```python
from build123d import *

# Parameters (mm, degrees)
SKETCH1_R                = 6.5
BOSS_EXTRUDE1_DEPTH      = 20
SKETCH2_R                = 6.45
BOSS_EXTRUDE2_DEPTH      = 9
SKETCH3_R                = 4
BOSS_EXTRUDE3_DEPTH      = 3
SKETCH4_RX               = 10
SKETCH4_RY               = 8
BOSS_EXTRUDE4_DEPTH      = 4
BOSS_EXTRUDE4_DEPTH_BACK = 4
FILLET2_R                = 1
SKETCH5_R                = 2
BOSS_EXTRUDE5_DEPTH      = 11.5
SKETCH8_R                = 2.5
CUT_EXTRUDE1_DEPTH       = 11.5
SKETCH9_R                = 6.45
BOSS_EXTRUDE6_DEPTH      = 60
SKETCH10_R               = 2
CUT_EXTRUDE2_DEPTH       = 10
SKETCH11_R               = 3.674860137
SKETCH11_R_2             = 2
BOSS_EXTRUDE7_DEPTH      = 1


with BuildPart() as part:
    # Sketch1 → Boss-Extrude1 (new body)
    with BuildSketch(Plane(origin=(0, 0, 0), x_dir=(0, 0, -1), z_dir=(1, 0, 0))):
        Circle(SKETCH1_R)
    extrude(amount=BOSS_EXTRUDE1_DEPTH)

    # Sketch2 → Boss-Extrude2 (add)
    with BuildSketch(Plane(origin=(20, 0, 0), x_dir=(0, 0, -1), z_dir=(1, 0, 0))):
        Circle(SKETCH2_R)
    extrude(amount=BOSS_EXTRUDE2_DEPTH)

    # Sketch3 → Boss-Extrude3 (add)
    with BuildSketch(Plane(origin=(29, 0, 0), x_dir=(0, 0, -1), z_dir=(1, 0, 0))):
        Circle(SKETCH3_R)
    extrude(amount=BOSS_EXTRUDE3_DEPTH)



with BuildPart() as body_2:
    # Sketch4 → Boss-Extrude4 (new body, two sides)
    with BuildSketch(Plane.XY) as boss_extrude4_sk:
        with Locations(Location((45.959697712, 0), (0, 0, 180))):
            Ellipse(SKETCH4_RX, SKETCH4_RY)
    extrude(amount=BOSS_EXTRUDE4_DEPTH)
    extrude(boss_extrude4_sk.sketch, amount=-BOSS_EXTRUDE4_DEPTH_BACK)

    # Fillet2
    fillet2_edges = [body_2.edges().sort_by_distance(p)[0] for p in [
        (55.959697589, 0.00125173, 4),
        (55.959697589, 0.00125173, -4),
    ]]
    fillet(fillet2_edges, radius=FILLET2_R)


with BuildPart() as part_1:
    add(part.part)

    add(body_2.part)  # Boss-Extrude5 merges body 2
    # Sketch5 → Boss-Extrude5 (add)
    with BuildSketch(Plane(origin=(32, 0, 0), x_dir=(0, 0, -1), z_dir=(1, 0, 0))):
        Circle(SKETCH5_R)
    extrude(amount=BOSS_EXTRUDE5_DEPTH)

    # Sketch8 → Cut-Extrude1 (cut, through all)
    with BuildSketch(Plane.XY.offset(4)):
        with Locations((45.959697644, 0)):
            Circle(SKETCH8_R)
    extrude(amount=-CUT_EXTRUDE1_DEPTH, mode=Mode.SUBTRACT)

    # Sketch9 → Boss-Extrude6 (add)
    with BuildSketch(Plane.ZY):
        Circle(SKETCH9_R)
    extrude(amount=BOSS_EXTRUDE6_DEPTH)

    # Sketch10 → Cut-Extrude2 (cut)
    with BuildSketch(Plane.ZY.offset(60)):
        Circle(SKETCH10_R)
    extrude(amount=-CUT_EXTRUDE2_DEPTH, mode=Mode.SUBTRACT)

    # Sketch11 → Boss-Extrude7 (add)
    with BuildSketch(Plane.ZY.offset(60)):
        Circle(SKETCH11_R)
        Circle(SKETCH11_R_2, mode=Mode.SUBTRACT)
    extrude(amount=BOSS_EXTRUDE7_DEPTH)


solid = part_1.part
```
CAD build for the part. Positions are in the model's coordinates, mm. A direction names the side the tool comes from. Round coordinates to 2 decimals unless told otherwise and drop trailing zeros. Order: outer loops, then holes, each group sorted by start corner. A loop starts at its lowest first (then second) coordinate and runs counter-clockwise, first axis right, second up. Notation, with made-up numbers: (33, 28.5) -> (57, 28.5) arc R18 cw to (57, 53.5) -> close; hole circle Ø11 at (84.25, 58.5). An arc over 180 degrees is marked (long way). One line per question, with ' | ' between items.
Q1. Drop flat-ended pins along their axis: pin 1 (3 mm diameter, centred on x = -27.5, z = -2, fed in from +Y); pin 2 (1.5 mm diameter, centred on x = -36.5, y = 2, fed in from +Z); pin 3 (1 mm diameter, centred on x = 12, y = -5.5, fed in from +Z). Give the stop position or say it passes through.
Completed:
pin 1: stops at y = 6.43 | pin 2: stops at z = 6.33 | pin 3: stops at z = 4.15
Q2. Slice it at A-A (x = -4.5). Write the cut outline in (y, z), then the cut area to 3 significant figures.
Completed:
outline: circle Ø12.9 at (0, 0) | area: 131 mm^2
Q3. Probe probe 1 along X at (y, z) = (-0.25, -2.25); probe 2 along Y at (x, z) = (-55.75, 0); probe 3 along X at (y, z) = (1.25, -2.5). List the from-to ranges inside material, lowest first.
Completed:
probe 1: x = -61 to 32, 35.96 to 43.47, 48.45 to 55.95 | probe 2: y = -6.45 to -2, 2 to 6.45 | probe 3: x = -61 to 32, 36.08 to 43.79, 48.12 to 55.84
Q4. Which spindle directions (+Z, -Z, +X, -X, +Y, -Y) get a long thin tool onto all of the face, cutting with end or side? Do faces 1 (the flat face through (-61, -2, 2)), 2 (the flat face through (48, 2, 4)), 3 (the cylindrical face through (-29.58, -6.297, -1.398)), 4 (the flat face through (32, -1, 2)). Say none if no direction does.
Completed:
face 1: +Z, -Z, -X, +Y, -Y | face 2: +Z, +X, +Y, -Y | face 3: -X | face 4: none
Q5. Two-plate mould, pull along Y, no slides. Class faces 5 (the cylindrical face through (-55, -2, 0)), 6 (the cylindrical face through (24.437, -6.297, 1.398)), 7 (the cylindrical face through (43.462, 0.11, 0.056)), 8 (the flat face through (48, 2, -4)): released by +Y, released by -Y, zero draft, split by the parting line, or undercut.
Completed:
face 5: undercut | face 6: split by the parting line | face 7: undercut | face 8: zero draft
